Could you check a few things on this model? Use its own coordinates, in mm. Face numbers are marked on the shaded views. A direction names the side the tool comes from. Round coordinates to 2 decimals unless told otherwise and drop trailing zeros. Order: outer loops, then holes, each group sorted by start corner. A loop starts at its lowest first (then second) coordinate and runs counter-clockwise, first axis right, second up. Notation, with made-up numbers: (87.25, -25.5) - (121.25, -25.5) arc R14 ccw to (121.25, -16.5) - close; hole circle Ø10 at (51.5, -28.75). An arc over 180 degrees is marked (long way). Use one line per item in the form item = value.
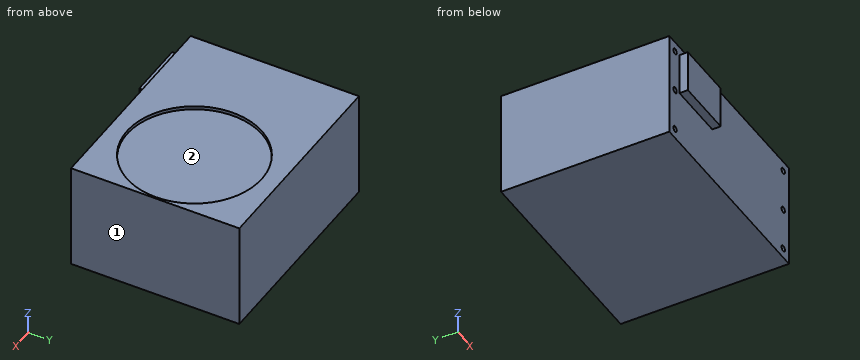
from build123d import *

# Parameters (mm, degrees)
F0_W     = 125
F0_H     = 63.5
F0_R     = 1.755
F0_W_2   = 34.3037378043
F0_H_2   = 25.238768314
F1_DEPTH = 100
F2_DEPTH = 5
F3_DEPTH = 5
F4_R     = 40
F5_DEPTH = 2


# Not quite as in the source:
# - a feature names something its author has since deleted; it is built from what else it names


with BuildPart() as f1:
    # F0 (on Front) → F1 (new body)
    with BuildSketch(Plane.XZ):
        Rectangle(F0_W, F0_H)
        with Locations((-56.5, -25.75)):
            Circle(F0_R, mode=Mode.SUBTRACT)
        with Locations((56.5, -25.75)):
            Circle(F0_R, mode=Mode.SUBTRACT)
        with Locations((-56.5, 0)):
            Circle(F0_R, mode=Mode.SUBTRACT)
        with Locations((-34.777761437, 13.8649413711)):
            Rectangle(F0_W_2, F0_H_2, mode=Mode.SUBTRACT)
        with Locations((-56.5, 25.75)):
            Circle(F0_R, mode=Mode.SUBTRACT)
        with Locations((56.5, 0)):
            Circle(F0_R, mode=Mode.SUBTRACT)
        with Locations((56.5, 25.75)):
            Circle(F0_R, mode=Mode.SUBTRACT)
        with Locations((-34.777761437, 13.8649413711)):
            Rectangle(F0_W_2, F0_H_2)
        with Locations((-56.5, 25.75)):
            Circle(F0_R)
        with Locations((-56.5, 0)):
            Circle(F0_R)
        with Locations((-56.5, -25.75)):
            Circle(F0_R)
        with Locations((56.5, -25.75)):
            Circle(F0_R)
        with Locations((56.5, 0)):
            Circle(F0_R)
        with Locations((56.5, 25.75)):
            Circle(F0_R)
    extrude(amount=-F1_DEPTH)

    # F0 (on Front) → F2 (join)
    with BuildSketch(Plane.XZ):
        with Locations((-34.777761437, 13.8649413711)):
            Rectangle(F0_W_2, F0_H_2)
    extrude(amount=F2_DEPTH)

    # F0 (on Front) → F3 (cut)
    with BuildSketch(Plane.XZ):
        with Locations((-56.5, 25.75)):
            Circle(F0_R)
        with Locations((-56.5, 0)):
            Circle(F0_R)
        with Locations((-56.5, -25.75)):
            Circle(F0_R)
        with Locations((56.5, -25.75)):
            Circle(F0_R)
        with Locations((56.5, 0)):
            Circle(F0_R)
        with Locations((56.5, 25.75)):
            Circle(F0_R)
    extrude(amount=-F3_DEPTH, mode=Mode.SUBTRACT)

    # F4 (on face) → F5 (cut)
    with BuildSketch(Plane.XY.offset(31.75)):
        with Locations((21.5, 50)):
            Circle(F4_R)
    extrude(amount=-F5_DEPTH, mode=Mode.SUBTRACT)


solid = f1.part
Item 1: Will these pins go through, and if not, where does the flat tip stop? P1, Ø3, axis at x = 57, z = 25.5, coming from the -Y side; P2, Ø2.5, axis at x = -38, y = -1.5, coming from the -Z side; P3, Ø24, axis at x = 16.5, y = 68, coming from the +Z side.
Found:
P1 = 0
P2 = 1.25
P3 = 29.75
Item 2: For the marked faces 1 and 2, which set-ups out of +Z, -Z, +X, -X, +Y, -Y let a thin tool reach every point of the face, with its end or its side?
Found:
face_1 = +Z, -Z, +X, +Y, -Y
face_2 = +Z
Item 3: Imagine slicing it at B-B on y = 50. Please give me the cut outline in (x, z), plus the area to 3 significant figures.
Found:
outline = (-62.5, -31.75) - (62.5, -31.75) - (62.5, 31.75) - (61.5, 31.75) - (61.5, 29.75) - (-18.5, 29.75) - (-18.5, 31.75) - (-62.5, 31.75) - close
area = 7,780 mm2
Item 4: I need wall thicknesses on L1, parallel to Z at x = -56.5, y = 2.4 (3 decimals); L2, parallel to Y at x = 21, z = 30; L3, parallel to X at y = 1, z = -25. Which ranges of each line are inside material? Lowest first, please.
Found:
L1 = -31.75 to -27.505, -23.995 to -1.755, 1.755 to 23.995, 27.505 to 31.75
L2 = 0 to 10, 90 to 100
L3 = -62.5 to -58.09, -54.91 to 54.91, 58.09 to 62.5
Item 5: Imagine slicing it at A-A on z = -25.75. Please give me the cut outline in (x, y) (3 decimals).
Found:
outline = (-62.5, 0) - (-58.255, 0) - (-58.255, 5) - (-54.745, 5) - (-54.745, 0) - (54.745, 0) - (54.745, 5) - (58.255, 5) - (58.255, 0) - (62.5, 0) - (62.5, 100) - (-62.5, 100) - close
Item 6: Imagine slicing it at C-C on x = -29. Please give me the cut outline in (y, z).
Found:
outline = (-5, 1.25) - (0, 1.25) - (0, -31.75) - (100, -31.75) - (100, 31.75) - (0, 31.75) - (0, 26.48) - (-5, 26.48) - close
Item 7: Imagine slicing it at D-D on z = -19. Please give me the cut outline in (x, y).
Found:
outline = (-62.5, 0) - (62.5, 0) - (62.5, 100) - (-62.5, 100) - close
